Verification items for the finished model (mm, model axes). Face numbers are marked on the shaded views. A direction names the side the tool comes from. Give positions to 0.01 mm unless a question says otherwise; leave off trailing zeros. Order: outer loops, then holes, each group sorted by start corner. A loop starts at its lowest first (then second) coordinate and runs counter-clockwise, first axis right, second up. Notation, with made-up numbers: (46.5, 64) - (58.5, 64) arc R17 ccw to (58.5, 69) - close; hole circle Ø1 at (33.5, 63.5). An arc over 180 degrees is marked (long way). Answer as a JSON object with one key per item and string values. Group by question number.
(1) Section check A-A (y = 30.5). Record the boundary of the cut face in (x, z).
(2) Mould release check, pull along X, two halves, no side actions. Record for the marked faces 4, 5 and 6: +X half, -X half, draft (parallel to the pull), parting line (faces both ways), or undercut.
(3) Depth check by flat-ended pin: pin 1 Ø6 at (x, y) = (9.5, 35.5) entering from +Z; pin 2 Ø8 at (y, z) = (9, 20) entering from +X; pin 3 Ø6 at (x, z) = (-14.5, 21) entering from +Y. Enter the tip coordinate at first touch or a pass-through.
(4) Section check C-C (x = -5). Record the boundary of the cut face in (y, z), then the cut area to 3 significant figures.
(5) Access from +Z, -Z, +X, -X, +Y, -Y to the whole of each face (thin tool, end or side, straight path). Record for the marked faces 1, 2 and 3.
(6) Section check D-D (x = -14). Record the boundary of the cut face in (y, z).
(7) Thickness scan on line 1 (X direction, y = 42.5, z = 21); line 2 (Z direction, x = 9, y = 36.5); line 3 (Y direction, x = 13, z = 15.75). Record the ranges inside material, lowest first.
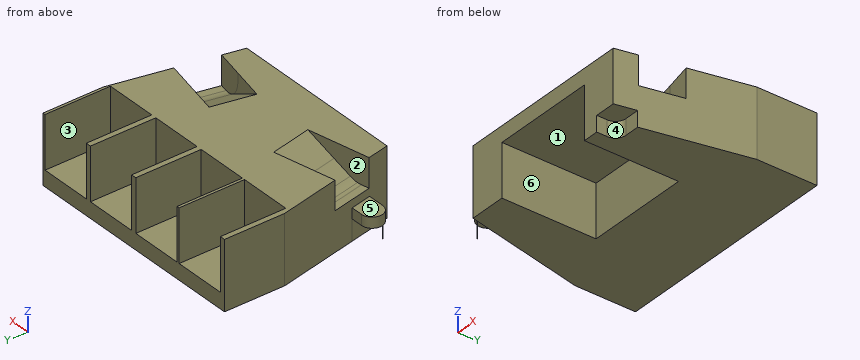
```python
from build123d import *

# Parameters (mm, degrees)
EXTRUDE_1_DEPTH      = 26
SKETCH_3_W           = 40
SKETCH_3_H           = 36
CUT_EXTRUDE_4_DEPTH  = 20
SKETCH_4_W           = 20
SKETCH_4_H           = 20
CUT_EXTRUDE_5_DEPTH  = 25
CUT_EXTRUDE_3_DEPTH  = 8
CUT_EXTRUDE_6_DEPTH  = 8
CUT_EXTRUDE_7_DEPTH  = 16
CUT_EXTRUDE_8_DEPTH  = 16
CUT_EXTRUDE_10_DEPTH = 6
EXTRUDE_3_DEPTH      = 12
CUT_EXTRUDE_11_DEPTH = 8


with BuildPart() as part:
    # 草图1 → 凸台-拉伸1 (new body)
    with BuildSketch(Plane.XY):
        Polygon((-34, -24), (34, -24), (44, 23), (44, 46), (-44, 46), (-44, 23), align=None)
    extrude(amount=EXTRUDE_1_DEPTH)

    # 草图3 → 切除-拉伸4 (cut)
    with BuildSketch(Plane(origin=(0, 0, 0), x_dir=(-1, 0, 0), z_dir=(0, 0, -1))):
        with Locations((0, -6)):
            Rectangle(SKETCH_3_W, SKETCH_3_H)
    extrude(amount=-CUT_EXTRUDE_4_DEPTH, mode=Mode.SUBTRACT)

    # 草图4 → 切除-拉伸5 (cut)
    with BuildSketch(Plane(origin=(0, 46, 0), x_dir=(1, 0, 0), z_dir=(0, 1, 0))):
        with Locations((33, -16)):
            Rectangle(SKETCH_4_W, SKETCH_4_H)
        with Locations((11, -16)):
            Rectangle(SKETCH_4_W, SKETCH_4_H)
        with Locations((-11, -16)):
            Rectangle(SKETCH_4_W, SKETCH_4_H)
        with Locations((-32, -16)):
            Rectangle(SKETCH_4_W, SKETCH_4_H)
    extrude(amount=-CUT_EXTRUDE_5_DEPTH, mode=Mode.SUBTRACT)

    # Sketch 3D_5 → 切除-拉伸3 (cut, symmetric)
    with BuildSketch(Plane(origin=(-26.633413551, -5.666683734, 23.004025099), x_dir=(-0.691625335103945, -0.14715432661786076, 0.7071067811865475), z_dir=(-0.2081076444648591, 0.9781059289848354, 0))):
        with BuildLine():
            Line((0, 0), (5.656854249, 5.656854249))
            Line((5.656854249, 5.656854249), (11.313708499, 0))
            ThreePointArc((11.313708499, 0), (5.656854249, -13.656854249), (0, 0))
        make_face()
    extrude(amount=CUT_EXTRUDE_3_DEPTH, both=True, mode=Mode.SUBTRACT)

    # Sketch 3D_6 → 切除-拉伸6 (cut, symmetric)
    with BuildSketch(Plane(origin=(34.478414998, -7.335832978, 14.99907516), x_dir=(0.5895982688198705, -0.12544644017993214, 0.7978954016979886), z_dir=(-0.20810764446495697, -0.9781059289848145, -6.6559639472978385e-12))):
        with BuildLine():
            Line((0, 0), (6.376045072, -8.439700449))
            Line((6.376045072, -8.439700449), (17.547318622, 0))
            Line((17.547318622, 0), (11.17127355, 8.439700449))
            Line((11.17127355, 8.439700449), (6.348906145, 14.822863662))
            Line((6.348906145, 14.822863662), (1.560795809, 11.205530619))
            ThreePointArc((1.560795809, 11.205530619), (-1.540343474, 5.926016705), (0, 0))
        make_face()
    extrude(amount=CUT_EXTRUDE_6_DEPTH, both=True, mode=Mode.SUBTRACT)

    # 草图7 → 切除-拉伸7 (cut)
    with BuildSketch(Plane(origin=(-1.664861156, 7.824847432, 0), x_dir=(0.9781059289848355, 0.2081076444648587, 0), z_dir=(0.2081076444648587, -0.9781059289848355, 0))):
        with BuildLine():
            Line((-24.556702047, 20), (-31.200844281, 16.10051891))
            ThreePointArc((-31.200844281, 16.10051891), (-33.152072653, 15.280030806), (-35.250185053, 15))
            Line((-35.250185053, 15), (-43.250185053, 15))
            Line((-43.250185053, 15), (-43.250185053, 23))
            ThreePointArc((-43.250185053, 23), (-40.3181561, 29.189965223), (-33.671267687, 30.842641134))
            Line((-33.671267687, 30.842641134), (-10.087245225, 28.492198282))
            Line((-10.087245225, 28.492198282), (-24.556702047, 20))
        make_face()
    extrude(amount=CUT_EXTRUDE_7_DEPTH, mode=Mode.SUBTRACT)

    # 草图11 → 切除-拉伸8 (cut)
    with BuildSketch(Plane(origin=(-1.664861156, -7.824847432, 0), x_dir=(0.9781059289845859, -0.2081076444660318, -1.1269708570671002e-12), z_dir=(0.20810764446603178, 0.9781059289845858, 5.296763028184159e-12))):
        with BuildLine():
            Line((31.200844283, -16.100518909), (14.333584528, -26))
            Line((14.333584528, -26), (32.666556858, -30.571318601))
            ThreePointArc((32.666556858, -30.571318601), (42.196349228, -26.968728166), (40.460809076, -16.92962956))
            Line((40.460809076, -16.92962956), (38.250185053, -14.99907516))
            Line((38.250185053, -14.99907516), (35.250185053, -15))
            ThreePointArc((35.250185053, -15), (33.152072655, -15.280030806), (31.200844283, -16.100518909))
        make_face()
    extrude(amount=CUT_EXTRUDE_8_DEPTH, mode=Mode.SUBTRACT)

    # 草图12 → 切除-拉伸10 (cut)
    with BuildSketch(Plane(origin=(0, 0, 0), x_dir=(-1, 0, 0), z_dir=(0, 0, -1))):
        with BuildLine():
            Line((-34, -24), (-26, -24))
            Line((-26, -24), (-26, -20))
            ThreePointArc((-26, -20), (-27.171572875, -17.171572875), (-30, -16))
            Line((-30, -16), (-34, -16))
            Line((-34, -16), (-39.007185212, -16))
            Line((-39.007185212, -16), (-39.007185212, -24))
            Line((-39.007185212, -24), (-34, -24))
        make_face()
    extrude(amount=-CUT_EXTRUDE_10_DEPTH, mode=Mode.SUBTRACT)

    # 草图13 → 凸台-拉伸3 (add)
    with BuildSketch(Plane(origin=(0, 0, 0), x_dir=(-1, 0, 0), z_dir=(0, 0, -1))):
        with BuildLine():
            Line((34, -16), (42, -16))
            ThreePointArc((42, -16), (46, -12), (42, -8))
            Line((42, -8), (38, -8))
            Line((38, -8), (34, -8))
            Line((34, -8), (34, -16))
        make_face()
    extrude(amount=-EXTRUDE_3_DEPTH)

    # 草图14 → 切除-拉伸11 (cut)
    with BuildSketch(Plane(origin=(0, 0, 0), x_dir=(-1, 0, 0), z_dir=(0, 0, -1))):
        Polygon((37.404255319, -8), (51.058505752, -8), (50.951803073, -15.80656107), (42, -16), (35.70212766, -16), align=None)
    extrude(amount=-CUT_EXTRUDE_11_DEPTH, mode=Mode.SUBTRACT)


solid = part.part
```
Solutions:
{
 "1": {"outline": "(-44, 0) - (44, 0) - (44, 26) - (43, 26) - (43, 6) - (23, 6) - (23, 26) - (21, 26) - (21, 6) - (1, 6) - (1, 26) - (-1, 26) - (-1, 6) - (-21, 6) - (-21, 26) - (-22, 26) - (-22, 6) - (-42, 6) - (-42, 26) - (-44, 26) - close"},
 "2": {"face 4": "+X half", "face 5": "draft", "face 6": "undercut"},
 "3": {"pin 1": "stops at z = 6", "pin 2": "stops at x = 41.87", "pin 3": "stops at y = 21"},
 "4": {"outline": "(-24, 20) - (12, 20) - (12, 0) - (46, 0) - (46, 6) - (21, 6) - (21, 26) - (-24, 26) - close", "area": "600 mm2"},
 "5": {"face 1": "-Z, -Y", "face 2": "+Z, -X", "face 3": "+Z, +Y"},
 "6": {"outline": "(-24, 20) - (12, 20) - (12, 0) - (46, 0) - (46, 6) - (21, 6) - (21, 26) - (-3.08, 26) - (-11.16, 25.01) - (-11.16, 26) - (-24, 26) - close"},
 "7": {"line 1": "x = -44 to -42, -22 to -21, -1 to 1, 21 to 23, 43 to 44", "line 2": "z = 0 to 6", "line 3": "y = 12 to 21"}
}
